from build123d import *

# Parameters (mm, degrees)
SKETCH1_W                                           = 152.4
SKETCH1_H                                           = 101.6
BOSS_EXTRUDE1_DEPTH                                 = 16.002
CBORE_FOR_0_BINDING_HEAD_MACHINE_SCREW1_D           = 11.9126
CBORE_FOR_0_BINDING_HEAD_MACHINE_SCREW1_CBORE_D     = 19.05
CBORE_FOR_0_BINDING_HEAD_MACHINE_SCREW1_CBORE_DEPTH = 9.652
BOSS_EXTRUDE2_DEPTH                                 = 15.875
SKETCH8_R                                           = 9.525
CUT_EXTRUDE1_DEPTH                                  = 147.561301523


with BuildPart() as part:
    # Sketch1 → Boss-Extrude1 (new body)
    with BuildSketch(Plane(origin=(0, 0, 0), x_dir=(1, 0, 0), z_dir=(0, 1, 0))):
        Rectangle(SKETCH1_W, SKETCH1_H)
    extrude(amount=BOSS_EXTRUDE1_DEPTH)

    # CBORE for #0 Binding Head Machine Screw1 (through all)
    with Locations(Plane(origin=(0, 16.002, 0), x_dir=(1, 0, 0), z_dir=(0, 1, 0))):
        with Locations((-50.8, 0), (50.8, 0)):
            CounterBoreHole(CBORE_FOR_0_BINDING_HEAD_MACHINE_SCREW1_D / 2, CBORE_FOR_0_BINDING_HEAD_MACHINE_SCREW1_CBORE_D / 2, CBORE_FOR_0_BINDING_HEAD_MACHINE_SCREW1_CBORE_DEPTH)

    # Sketch7 → Boss-Extrude2 (add)
    with BuildSketch(Plane.XY.offset(50.8)):
        with BuildLine():
            Line((-25.4, 16.002), (-25.4, 47.752))
            ThreePointArc((-25.4, 47.752), (0, 73.152), (25.4, 47.752))
            Line((25.4, 47.752), (25.4, 16.002))
            Line((25.4, 16.002), (-25.4, 16.002))
        make_face()
    boss_extrude2 = extrude(amount=-BOSS_EXTRUDE2_DEPTH)

    # Mirror1: Boss-Extrude2 across plane
    add(boss_extrude2.mirror(Plane.XY))

    # Sketch8 → Cut-Extrude1 (cut, through all)
    with BuildSketch(Plane.XY.offset(50.8)):
        with Locations((0, 47.752)):
            Circle(SKETCH8_R)
    extrude(amount=-CUT_EXTRUDE1_DEPTH, mode=Mode.SUBTRACT)


solid = part.part
Source: CAD feature listing. Evaluate the final solid. Frame: model axes, mm. A direction names the side the tool comes from. Give positions to 0.01 mm unless a question says otherwise; leave off trailing zeros. Write each loop counter-clockwise with the first axis right and the second up, starting at its lowest first coordinate (ties: lowest second). Pieces come first, ordered by that corner, then holes. Notation, with made-up numbers: M 4.25,-25.5 L 45.25,-25.5 A22 cw 45.25,13.5 Z; hole C -6.5,70 d5. An arc over 180 degrees is marked long. Return JSON: item names as keys, results as strings. Group by question number.
1) Material intervals for line 1 along Z through (x, y) = (-50.8, 8.75) (3 decimals); line 2 along Y through (x, z) = (0, -46.25); line 3 along Z through (x, y) = (-10, 66) (3 decimals), sorted ascending. Write a range as [from, to].
2) Cut plane A-A, the plane x = 0. Output: boundary loops of the cut face in (y, z) (3 decimals), plus the area to 3 significant figures.
3) Set-up query: faces 1 (the face through (59.6, 11.24, 3.65)), 2 (the face through (-25.4, 32, -43)), 3 (the face through (25.4, 32, 43)). Return all of +Z, -Z, +X, -X, +Y, -Y with unobstructed straight access to the full face (end or side cutting, diameter ignored); none if empty.
4) Cut plane C-C, the plane y = 31.5. Output: boundary loops of the cut face in (x, z) (3 decimals).
5) Cut plane D-D, the plane x = -50.8. Output: boundary loops of the cut face in (y, z) (3 decimals), plus the area to 3 significant figures.
6) Pull-direction query (Z, two-part tool) for faces 4 (the face through (-5, 39, -34.925)), 5 (the face through (-76.2, 8, 1)), 6 (the face through (-1, 20, -50.8)); classes: pulls with the +Z half, pulls with the -Z half, needs draft (parallel to the pull), parting line crosses it, or undercut.
7) Pin query (flat end, axial travel): P1, Ø21, axis at x = 53.5, z = 1.5, coming from the +Y side; P2, Ø8, axis at y = 28, z = 41.5, coming from the -X side; P3, Ø12.5, axis at y = 38.5, z = -45.5, coming from the +X side. Return the tip coordinate at first contact, or that it passes through.
8) Cut plane B-B, the plane z = 0. Output: boundary loops of the cut face in (x, y) (3 decimals).
Recorded:
{
 "1": {"line 1": "z = [-50.8, -9.525], [9.525, 50.8]", "line 2": "y = [0, 38.23], [57.28, 73.15]", "line 3": "z = [-50.8, -34.925], [34.925, 50.8]"},
 "2": {"outline": "M 0,-50.8 L 38.227,-50.8 L 38.227,-34.925 L 16.002,-34.925 L 16.002,34.925 L 38.227,34.925 L 38.227,50.8 L 0,50.8 Z; M 57.277,-50.8 L 73.152,-50.8 L 73.152,-34.925 L 57.277,-34.925 Z; M 57.277,34.925 L 73.152,34.925 L 73.152,50.8 L 57.277,50.8 Z", "area": "2,840 mm²"},
 "3": {"face 1": "+Y", "face 2": "+Z, -Z, -X, +Y", "face 3": "+Z, -Z, +X, +Y"},
 "4": {"outline": "M -25.4,-50.8 L 25.4,-50.8 L 25.4,-34.925 L -25.4,-34.925 Z; M -25.4,34.925 L 25.4,34.925 L 25.4,50.8 L -25.4,50.8 Z"},
 "5": {"outline": "M 0,-50.8 L 16.002,-50.8 L 16.002,-9.525 L 6.35,-9.525 L 6.35,-5.956 L 0,-5.956 Z; M 0,5.956 L 6.35,5.956 L 6.35,9.525 L 16.002,9.525 L 16.002,50.8 L 0,50.8 Z", "area": "1,370 mm²"},
 "6": {"face 4": "undercut", "face 5": "needs draft", "face 6": "pulls with the -Z half"},
 "7": {"P1": "stops at y = 16", "P2": "stops at x = -25.4", "P3": "stops at x = 25.4"},
 "8": {"outline": "M -76.2,0 L -56.756,0 L -56.756,6.35 L -60.325,6.35 L -60.325,16.002 L -76.2,16.002 Z; M -44.844,0 L 44.844,0 L 44.844,6.35 L 41.275,6.35 L 41.275,16.002 L -41.275,16.002 L -41.275,6.35 L -44.844,6.35 Z; M 56.756,0 L 76.2,0 L 76.2,16.002 L 60.325,16.002 L 60.325,6.35 L 56.756,6.35 Z"}
}
